```python
from build123d import *

# Parameters (mm, degrees)
SKETCH_1_W          = 30.50790567
SKETCH_1_H          = 58.511029644
SKETCH_1_R          = 1.716069694
SKETCH_1_W_2        = 11.42456148
SKETCH_1_H_2        = 8.922497171
EXTRUDE_1_DEPTH     = 3.3
SKETCH_2_W          = 30.50790567
SKETCH_2_H          = 6
EXTRUDE_2_DEPTH     = 1
SKETCH_3_W          = 18.50790567
SKETCH_3_H          = 8
CUT_EXTRUDE_1_DEPTH = 3.3


with BuildPart() as part:
    # 草圖1 → 填料-伸長1 (new body)
    with BuildSketch(Plane.XY):
        with Locations((0, 11.421692739)):
            Rectangle(SKETCH_1_W, SKETCH_1_H)
        with Locations((-11.174415212, 10.166177917)):
            Circle(SKETCH_1_R, mode=Mode.SUBTRACT)
        with Locations((11.070768934, 10.080826612)):
            Circle(SKETCH_1_R, mode=Mode.SUBTRACT)
        with Locations((0, 23.470612751)):
            Rectangle(SKETCH_1_W_2, SKETCH_1_H_2, mode=Mode.SUBTRACT)
    extrude(amount=EXTRUDE_1_DEPTH)

    # 草圖2 → 填料-伸長2 (add)
    with BuildSketch(Plane.XY.offset(3.3)):
        with Locations((0, -0.833822083)):
            Rectangle(SKETCH_2_W, SKETCH_2_H)
        with Locations((0, -14.833822083)):
            Rectangle(SKETCH_2_W, SKETCH_2_H)
    extrude(amount=EXTRUDE_2_DEPTH)

    # 草圖3 → 除料-伸長1 (cut)
    with BuildSketch(Plane.XY.offset(3.3)):
        with Locations((0, -7.833822083)):
            Rectangle(SKETCH_3_W, SKETCH_3_H)
    extrude(amount=-CUT_EXTRUDE_1_DEPTH, mode=Mode.SUBTRACT)


solid = part.part
```
Part model, mm, in its own coordinate system. A direction names the side the tool comes from. Give positions to 0.01 mm unless a question says otherwise; leave off trailing zeros. Loops run counter-clockwise (first coordinate to the right, second up) from the corner with the lowest first, then second, coordinate; pieces in that order, holes last. Notation, with made-up numbers: M 37,-10.75 L 61,-10.75 A16 ccw 61,11.25 Z; hole C 24.25,86 d8. An arc over 180 degrees is marked long. Return JSON: item names as keys, results as strings.
1) Saw through at C-C, the plane x = -7. List the corners of the cut face in (y, z), then the cut area to 3 significant figures.
Calculated:
{"outline": "M -17.83,0 L -11.83,0 L -11.83,4.3 L -17.83,4.3 Z; M -3.83,0 L 40.68,0 L 40.68,3.3 L 2.17,3.3 L 2.17,4.3 L -3.83,4.3 Z", "area": "179 mm2"}
2) Saw through at A-A, the plane y = -9. List the corners of the cut face in (x, z).
Calculated:
{"outline": "M -15.25,0 L -9.25,0 L -9.25,3.3 L -15.25,3.3 Z; M 9.25,0 L 15.25,0 L 15.25,3.3 L 9.25,3.3 Z"}
3) Flat gauge pin, fed straight in: pin 1 Ø5 at (x, y) = (-2.5, 5.5) entering from +Z. Where does the tip first touch, or does it go through?
Calculated:
{"pin 1": "stops at z = 3.3"}
4) Saw through at B-B, the plane x = 0.5. List the corners of the cut face in (y, z).
Calculated:
{"outline": "M -17.83,0 L -11.83,0 L -11.83,4.3 L -17.83,4.3 Z; M -3.83,0 L 19.01,0 L 19.01,3.3 L 2.17,3.3 L 2.17,4.3 L -3.83,4.3 Z; M 27.93,0 L 40.68,0 L 40.68,3.3 L 27.93,3.3 Z"}
5) Saw through at D-D, the plane y = 22. List the corners of the cut face in (x, z).
Calculated:
{"outline": "M -15.25,0 L -5.71,0 L -5.71,3.3 L -15.25,3.3 Z; M 5.71,0 L 15.25,0 L 15.25,3.3 L 5.71,3.3 Z"}
6) Drill centre lines: line 1 (Y direction, x = 0.5, z = 3.2); line 2 (Y direction, x = 13, z = 4); line 3 (X direction, y = 26, z = 2.9). Where is each one in solid material? Low to high.
Calculated:
{"line 1": "y = -17.83 to -11.83, -3.83 to 19.01, 27.93 to 40.68", "line 2": "y = -17.83 to -11.83, -3.83 to 2.17", "line 3": "x = -15.25 to -5.71, 5.71 to 15.25"}
7) Pull direction Y, two halves, no side cores. Call faces 1 (the face through (15.254, 11, 2)), 2 (the face through (0, -17.834, 2)), 3 (the face through (-12.439, 11.326, 1.627)): released by +Y, released by -Y, zero draft, split by the parting line, or undercut.
Calculated:
{"face 1": "zero draft", "face 2": "released by -Y", "face 3": "undercut"}
8) 3-axis set-ups, long thin cutter, end or side, ignore diameter. For faces 4 (the face through (0, -3.834, 3)), 5 (the face through (-12, -8, 3.3)), 6 (the face through (0, 27.932, 2)), 7 (the face through (0, 17, 3.3)): which of +Z, -Z, +X, -X, +Y, -Y reach the whole face in a straight line?
Calculated:
{"face 4": "+Z", "face 5": "+Z, +X, -X", "face 6": "+Z, -Z", "face 7": "+Z, +X, -X, +Y"}
